Solid Edge part; units mm, degrees
sketch "Sketch1" plane through (0, 0, 0) normal (0, -1, 0) x (1, 0, 0)
  line L0 (14, -14) -> (14, 14)
  line L1 (14, 14) -> (-14, 14)
  line L2 (-14, 14) -> (-14, -14)
  line L3 (-14, -14) -> (14, -14)
extrude "Protrusion1" add sketch "Sketch1" along normal blind 6
sketch "Sketch2" plane through (0, -6, 0) normal (0, -1, 0) x (1, 0, 0)
  line L0 (16, 16) -> (-16, 16)
  line L1 (-16, 16) -> (-16, -16)
  line L2 (-16, -16) -> (16, -16)
  line L3 (16, -16) -> (16, 16)
extrude "ExtrudedProtrusion_2" add sketch "Sketch2" along normal blind 6
sketch "Sketch3" plane through (0, -9, 16) normal (0, 0, 1) x (-1, 0, 0)
  line L0 (16, 3) -> (16, -3)
  line L1 (16, -3) -> (-16, -3)
  line L2 (-16, -3) -> (-16, 3)
  line L3 (-16, 3) -> (16, 3)
extrude "ExtrudedProtrusion_3" add sketch "Sketch3" along normal blind 44.57
mirror "Mirror1" about plane through (0, -9, 60.57) normal (0, 0, 1) of "Protrusion1", "ExtrudedProtrusion_2", "ExtrudedProtrusion_3"
mirror "Mirror2" about plane through (0, -9, 60.57) normal (0, 0, 1) of "Protrusion1", "ExtrudedProtrusion_3", "ExtrudedProtrusion_2"
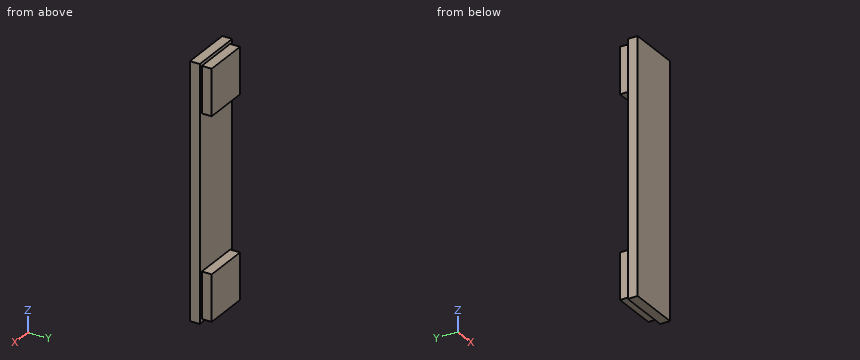
Geometry check sheet. Reference: the model listing, model coordinates, mm. Give positions to 0.01 mm unless a question says otherwise; leave off trailing zeros. Write each loop counter-clockwise with the first axis right and the second up, starting at its lowest first coordinate (ties: lowest second). Pieces come first, ordered by that corner, then holes. Notation, with made-up numbers: (74, -26) - (104, -26) arc R18 cw to (104, -21) - close; hole circle Ø6 at (48, 69). An arc over 180 degrees is marked (long way). Use a Markdown table: item, result.
Q1. Section check A-A, the plane y = -3. Enter the section's corners in (x, z), then the cut area to 3 significant figures.
Computed:
| item | result |
|---|---|
| outline | (-14, -14) - (14, -14) - (14, 14) - (-14, 14) - close; (-14, 107.14) - (14, 107.14) - (14, 135.14) - (-14, 135.14) - close |
| area | 1,570 mm² |
Q2. Thickness scan on L1, parallel to Z at x = -13.5, y = -3.25; L2, parallel to Y at x = -13.5, z = 73; L3, parallel to X at y = -2.75, z = 113. Record the ranges inside material, lowest first. Write a range as [from, to].
Computed:
| item | result |
|---|---|
| L1 | z = [-14, 14], [107.14, 135.14] |
| L2 | y = [-12, -6] |
| L3 | x = [-14, 14] |
Q3. Section check B-B, the plane x = 0.5. Enter the section's corners in (y, z), then the cut area to 3 significant figures.
Computed:
| item | result |
|---|---|
| outline | (-12, -16) - (-6, -16) - (-6, -14) - (0, -14) - (0, 14) - (-6, 14) - (-6, 107.14) - (0, 107.14) - (0, 135.14) - (-6, 135.14) - (-6, 137.14) - (-12, 137.14) - close |
| area | 1,250 mm² |
Q4. Go/stop test with flat-tipped pins: P1, Ø3, axis at y = -2, z = -2.5, coming from the +X side; P2, Ø6.5, axis at y = -2.5, z = -2, coming from the -X side; P3, Ø1.8, axis at x = -2, y = -1.5, coming from the -Z side. Record where each tip stops, or that it passes through.
Computed:
| item | result |
|---|---|
| P1 | stops at x = 14 |
| P2 | stops at x = -14 |
| P3 | stops at z = -14 |
Q5. Section check D-D, the plane z = 82.5. Enter the section's corners in (x, y).
Computed:
| item | result |
|---|---|
| outline | (-16, -12) - (16, -12) - (16, -6) - (-16, -6) - close |
Q6. Section check C-C, the plane z = -1. Enter the section's corners in (x, y).
Computed:
| item | result |
|---|---|
| outline | (-16, -12) - (16, -12) - (16, -6) - (14, -6) - (14, 0) - (-14, 0) - (-14, -6) - (-16, -6) - close |
